Autodesk Inventor part; units mm, degrees
ref_plane "YZ Plane" through (0, 0, 0) normal (1, 0, 0) x (0, 1, 0)
ref_plane "XZ Plane" through (0, 0, 0) normal (0, 1, 0) x (-1, 0, 0)
ref_plane "XY Plane" through (0, 0, 0) normal (0, 0, 1) x (1, 0, 0)
sketch "Sketch5" plane through (0, 0, 0) normal (0, 1, 0) x (-1, 0, 0)
  circle A0 centre (0, 0) radius 1.75
  circle A1 centre (0, 0) radius 24
  line L0 (0, 0) -> (24, 0)
  line L1 (24, 0) -> (29, 0)
  line L2 (24, 0) -> (24, -5)
  line L3 (24, 0) -> (29, 0) construction
  line L4 (24, -5) -> (0, -5)
  line L5 (0, -5) -> (0, 5)
  line L6 (0, 5) -> (24, 5)
  line L7 (24, 5) -> (24, -5)
  line L8 (-7.6699, 23.2846) -> (4.3301, 2.5)
  line L9 (-4.3301, -2.5) -> (-16.3301, 18.2846)
  line L10 (4.3301, 2.5) -> (-4.3301, -2.5)
  line L11 (-12, 20.7846) -> (-7.6699, 23.2846)
  line L12 (-16.3301, 18.2846) -> (-7.6699, 23.2846)
  line L13 (-16.3301, -18.2846) -> (-4.3301, 2.5)
  line L14 (4.3301, -2.5) -> (-7.6699, -23.2846)
  line L15 (-4.3301, 2.5) -> (4.3301, -2.5)
  line L16 (-12, -20.7846) -> (-16.3301, -18.2846)
  line L17 (-7.6699, -23.2846) -> (-16.3301, -18.2846)
  dimension "d78" = 48
  dimension "d54" = 3.5
  dimension "d82" = 5
  dimension "d83" = 5
  dimension "d84" = 90
  dimension "d85" = 24
  dimension "d86" = 10
  dimension "d89" = 360
extrude "Extrusion7" add sketch "Sketch5" along normal blind 10 contours L0 L10 A0 | L0 A1 L4 L14 L15 A0 | A0 L15 L0 | A0 L10 L8 L6 A1 L0 | L10 L5 A0 | A0 L5 L6 L8 L10 | L15 L14 L4 L5 A0 | A0 L5 L15 | L15 A0 L5 | L5 A0 L10 | L10 A0 L15 | L2 L4 A1 | A1 L6 L7 | A0 L15 L13 L9 A1 L8 L6 L5 | L5 L4 L14 A1 L13 L9 L10 A0 | L10 L9 L13 L15 A0 | A1 L11 L8 | L14 L17 A1 | A1 L9 L12 | L16 L13 A1
sketch "Sketch7" plane through (5.7735, 0, 0) normal (0.866, 0, 0.5) x (0.5, 0, -0.866)
  line L0 (21.1132, 0) -> (21.1132, 10)
  line L1 (21.1132, 10) -> (21.1132, 5)
  line L2 (21.1132, 5) -> (16.1132, 5)
  circle A0 centre (16.1132, 5) radius 1.5
  point P0 (-2.8868, 0)
  dimension "d93" = 5
  dimension "d94" = 5
  dimension "d95" = 3
extrude "Extrusion8" cut sketch "Sketch7" against normal blind 10
sketch "Sketch8" plane through (0, 10, 0) normal (0, 1, 0) x (1, 0, 0)
  circle A0 centre (0, 0) radius 1.75
  dimension "d98" = 3.5
extrude "Extrusion9" cut sketch "Sketch8" against normal blind 10
pattern_circular "Circular Pattern7" count 3 over 360 about axis through (0, 10, 0) along (0, -1, 0) of "Extrusion8"
fillet "Fillet7" radius 10 3 edges at (5.7735, 5, 0) (-2.8868, 5, 5) (-2.8868, 5, -5)
fillet "Fillet8" radius 2 23 edges at (7.6699, 5, 23.2846) (16.3301, 5, 18.2846) (-24, 5, 5) (-24, 10, 0) (16.3301, 5, -18.2846) (12, 10, -20.7846) (7.6699, 5, -23.2846) (-16.3301, 10, -5) (3.8349, 10, -16.6423) (12.4952, 10, 11.6423) (12.4952, 10, -11.6423) (-16.3301, 10, 5) (3.8349, 10, 16.6423) (-24, 5, -5) (-24, 0, 0) (12, 0, 20.7846) (12.4952, 0, -11.6423) (12.4952, 0, 11.6423) (-16.3301, 0, 5) (3.8349, 0, 16.6423) (-16.3301, 0, -5) (3.8349, 0, -16.6423) (12, 0, -20.7846)
properties part number "Custom_Delta_End_Effector"
For this review, take the finished solid that the model builds, in its own axes (mm). A direction names the side the tool comes from. Round coordinates to 2 decimals unless told otherwise and drop trailing zeros. Write each loop counter-clockwise with the first axis right and the second up, starting at its lowest first coordinate (ties: lowest second). Pieces come first, ordered by that corner, then holes. Notation, with made-up numbers: (22, 23.5) - (56, 23.5) arc R12 cw to (56, 41.5) - close; hole circle Ø11 at (-13, 43.5). An arc over 180 degrees is marked (long way). Put each result on its own line as item: value.
Q1. Wall thickness on probe 1 along X at (y, z) = (3, 0); probe 2 along X at (y, z) = (5.5, 0); probe 3 along Z at (x, y) = (8.5, 5.5): over which ranges is each line inside the solid? List them lowest first.
Solved:
probe 1: x = -24 to -1.75, 1.75 to 7.32
probe 2: x = -24 to -20.41, -17.59 to -1.75, 1.75 to 7.32
probe 3: z = -22.55 to -18.66, -15.4 to -4.71, 4.71 to 15.4, 18.66 to 22.55
Q2. We need section D-D (x = -11.5). Give the boundary of the cut face in (y, z).
Solved:
outline: (0, -3) arc R2 ccw to (2, -5) - (8, -5) arc R2 ccw to (10, -3) - (10, 3) arc R2 ccw to (8, 5) - (2, 5) arc R2 ccw to (0, 3) - close
Q3. We need section C-C (y = 7.5). Give the boundary of the cut face in (x, z), and give its area (3 significant figures).
Solved:
outline: (-24, -3) arc R2 ccw to (-22, -5) - (-8.66, -5) arc R10 cw to (0, -10) - (6.67, -21.55) arc R2 ccw to (9.4, -22.28) - (14.6, -19.28) arc R2 ccw to (15.33, -16.55) - (8.66, -5) arc R10 cw to (8.66, 5) - (15.33, 16.55) arc R2 ccw to (14.6, 19.28) - (9.4, 22.28) arc R2 ccw to (6.67, 21.55) - (0, 10) arc R10 cw to (-8.66, 5) - (-22, 5) arc R2 ccw to (-24, 3) - close; hole circle Ø3.5 at (0, 0)
area: 678 mm2
Q4. Machinability: for faces 1 (the face through (-15.24, 9.4, -4.43)), 2 (the face through (-15.42, 9.4, 4.43)), 3 (the face through (12.042, 4.958, -10.857)), which of the approach directions +Z, -Z, +X, -X, +Y, -Y give a long, thin tool a straight path to every point of the face, cutting with its end or side? Answer none if there is none.
Solved:
face 1: -Z, -X, +Y
face 2: +Z, -X, +Y
face 3: +X, +Y, -Y
Q5. Insertion check: pin 1 Ø5 at (y, z) = (2, -13.5) entering from -X; pin 2 Ø1 at (y, z) = (6, 9) entering from -X; pin 3 Ø5 at (x, y) = (-18, 5.5) entering from -Z. Each pin has a flat end and moves straight along its axis. Give the tip position at first contact, or say it passes through.
Solved:
pin 1: stops at x = 0.58
pin 2: stops at x = -1.06
pin 3: stops at z = -5
Q6. Mouldability with a two-part tool opening along Z and no side actions: class faces 4 (the face through (-23.4, 5.04, -4.43)), 5 (the face through (11.7, 0.6, 20.3)), 6 (the face through (15.524, 6.056, 18.091)), 7 (the face through (1, 0, 2)) as released by +Z, released by -Z, zero draft, split by the parting line, or undercut.
Solved:
face 4: released by -Z
face 5: released by +Z
face 6: undercut
face 7: zero draft
Q7. We need section A-A (z = 0). Give the boundary of the cut face in (x, y), and give its area (3 significant figures).
Solved:
outline: (-24, 2) arc R2 ccw to (-22, 0) - (-1.75, 0) - (-1.75, 10) - (-22, 10) arc R2 ccw to (-24, 8) - close; (1.75, 0) - (5.32, 0) arc R2 ccw to (7.32, 2) - (7.32, 8) arc R2 ccw to (5.32, 10) - (1.75, 10) - close; hole circle Ø3 at (-19, 5)
area: 268 mm2
Q8. We need section B-B (y = 5). Count the separate pieces of the cut face and the enclosed holes in it, and give its area (3 significant figures).
Solved:
separate pieces: 4
enclosed holes: 1
area: 588 mm2
